```python
from build123d import *

# Parameters (mm, degrees)
ESQUISSE1_R             = 40
BOSS_EXTRU_1_DEPTH      = 24
CONG_2_R                = 12
ESQUISSE2_R             = 28
ENL_V_MAT_EXTRU_1_DEPTH = 8
ENL_V_START             = -8
ESQUISSE3_R             = 28
ENL_V_MAT_EXTRU_2_DEPTH = 8
ESQUISSE4_R             = 3.5
ESQUISSE4_R_2           = 2
ENL_V_MAT_EXTRU_3_DEPTH = 59.787753895
BOSS_EXTRU_2_START      = 10
ESQUISSE5_R             = 28
ESQUISSE5_R_2           = 24.698706658
BOSS_EXTRU_2_DEPTH      = 10


with BuildPart() as part:
    # Esquisse1 → Boss.-Extru.1 (new body)
    with BuildSketch(Plane(origin=(0, 0, 0), x_dir=(1, 0, 0), z_dir=(0, 1, 0))):
        with Locations(Location((0, 0, 0), (0, 0, 270))):
            Circle(ESQUISSE1_R)
    extrude(amount=BOSS_EXTRU_1_DEPTH)

    # Congé2
    cong_2_edges = [part.edges().sort_by_distance(p)[0] for p in [
        (0, 0, -40),
        (0, 24, -40),
    ]]
    fillet(cong_2_edges, radius=CONG_2_R - 0.0001)  # a hair under: the kernel refuses the full size

    # Esquisse2 → Enlèv. mat.-Extru.1 (cut)
    with BuildSketch(Plane(origin=(0, 24, 0), x_dir=(1, 0, 0), z_dir=(0, 1, 0))):
        with Locations(Location((0, 0, 0), (0, 0, 270))):
            Circle(ESQUISSE2_R)
    extrude(amount=-ENL_V_MAT_EXTRU_1_DEPTH, mode=Mode.SUBTRACT)

    # Esquisse3 → Enlèv. mat.-Extru.2 (cut)
    with BuildSketch(Plane.XZ.offset(ENL_V_START)):
        with Locations(Location((0, 0, 0), (0, 0, 90))):
            Circle(ESQUISSE3_R)
    extrude(amount=ENL_V_MAT_EXTRU_2_DEPTH, mode=Mode.SUBTRACT)

    # Esquisse4 → Enlèv. mat.-Extru.3 (cut, through all)
    with BuildSketch(Plane(origin=(0, 16, 0), x_dir=(1, 0, 0), z_dir=(0, 1, 0))):
        with Locations(Location((0, 0, 0), (0, 0, 270))):
            Circle(ESQUISSE4_R)
        with Locations(Location((-2.866979911, 8.001901411, 0), (0, 0, 270))):
            Circle(ESQUISSE4_R_2)
        with Locations(Location((8.001901411, 2.866979911, 0), (0, 0, 270))):
            Circle(ESQUISSE4_R_2)
        with Locations(Location((2.866979911, -8.001901411, 0), (0, 0, 270))):
            Circle(ESQUISSE4_R_2)
        with Locations(Location((-8.001901411, -2.866979911, 0), (0, 0, 270))):
            Circle(ESQUISSE4_R_2)
        with Locations(Location((-6.408543331, 17.886603154, 0), (0, 0, 270))):
            Circle(ESQUISSE4_R)
        with Locations(Location((8.116213936, 17.179262829, 0), (0, 0, 270))):
            Circle(ESQUISSE4_R)
        with Locations(Location((17.886603154, 6.408543331, 0), (0, 0, 270))):
            Circle(ESQUISSE4_R)
        with Locations(Location((17.179262829, -8.116213936, 0), (0, 0, 270))):
            Circle(ESQUISSE4_R)
        with Locations(Location((6.408543331, -17.886603154, 0), (0, 0, 270))):
            Circle(ESQUISSE4_R)
        with Locations(Location((-8.116213936, -17.179262829, 0), (0, 0, 270))):
            Circle(ESQUISSE4_R)
        with Locations(Location((-17.886603154, -6.408543331, 0), (0, 0, 270))):
            Circle(ESQUISSE4_R)
        with Locations(Location((-17.179262829, 8.116213936, 0), (0, 0, 270))):
            Circle(ESQUISSE4_R)
    extrude(amount=-ENL_V_MAT_EXTRU_3_DEPTH, mode=Mode.SUBTRACT)

    # Esquisse5 → Boss.-Extru.2 (add)
    with BuildSketch(Plane(origin=(0, 16, 0), x_dir=(1, 0, 0), z_dir=(0, 1, 0)).offset(BOSS_EXTRU_2_START)):
        with Locations(Location((0, 0, 0), (0, 0, 90))):
            Circle(ESQUISSE5_R)
        with Locations(Location((0, 0, 0), (0, 0, 270))):
            Circle(ESQUISSE5_R_2, mode=Mode.SUBTRACT)
    extrude(amount=-BOSS_EXTRU_2_DEPTH)


solid = part.part
```
For this review, take the finished solid that the model builds, in its own axes (mm). A direction names the side the tool comes from. Coordinates: 2 decimals unless noted, no trailing zeros. Order: outer loops, then holes, each group sorted by start corner. A loop starts at its lowest first (then second) coordinate and runs counter-clockwise, first axis right, second up. Notation, with made-up numbers: (24.5, -20) - (52.5, -20) arc R15 ccw to (52.5, -3) - close; hole circle Ø1 at (-29.75, -3). An arc over 180 degrees is marked (long way). Answer as a JSON object with one key per item and string values. Group by question number.
1. We need section A-A on y = 13.75. Give the number of separate pieces and of enclosed holes in the cut face, then the cut area to 3 significant figures.
2. For probe 1 along Z at (x, y) = (-15.5, 9); probe 2 along Y at (x, z) = (-20.5, -16); probe 3 along Z at (x, y) = (7, 15.25), list the stretches that pass through material, from the lowest coordinate up.
3. The part is to be moulded in two halves that separate along Z. For faces 1 (the cylindrical face through (3.5, 12.1, 9.9)), 2 (the flat face through (25, 26, 0)), 3 (the cylindrical face through (27.334, 25.014, 6.07)), say which applies: pulls with the +Z half, pulls with the -Z half, needs draft (parallel to the pull), parting line crosses it, or undercut.
4. Clearance check with flat-ended pins moving along their axes: P1, Ø15, axis at x = 0, z = -2, coming from the +Y side; P2, Ø3, axis at x = -31.5, y = 18.5, coming from the -Z side; P3, Ø12, axis at y = 21, z = 6.5, coming from the +X side. State where each tip first meets the part, or that it passes through.
5. For faces 4 (the flat face through (0, 8, 6)), 5 (the cylindrical face through (24.489, 21.07, -3.215)), 6 (the cylindrical face through (6.05, 12.06, -3.3)), list the 3-axis set-ups (+Z, -Z, +X, -X, +Y, -Y) from which the entire face can be reached by the end or side of a thin tool; tool diameter is ignored.
6. We need section B-B on y = 4.5. State the section outline as (x, z) points.
Final values:
{
 "1": {"separate pieces": "1", "enclosed holes": "13", "area": "4,600 mm²"},
 "2": {"probe 1": "-36.46 to -11.19, -5.05 to 3.85, 8.97 to 36.46", "probe 2": "8 to 26", "probe 3": "-38.93 to -20.5, -13.86 to -4.6, -1.14 to 14.44, 21.34 to 38.93"},
 "3": {"face 1": "undercut", "face 2": "needs draft", "face 3": "parting line crosses it"},
 "4": {"P1": "y = 16", "P2": "z = -23.94", "P3": "x = 39.27"},
 "5": {"face 4": "-Y", "face 5": "+Y", "face 6": "+Y, -Y"},
 "6": {"outline": "circle Ø74.74 at (0, 0); hole circle Ø56 at (0, 0)"}
}
